Could you check a few things on this model? Use its own coordinates, in mm. A direction names the side the tool comes from. Coordinates: 2 decimals unless noted, no trailing zeros. Order: outer loops, then holes, each group sorted by start corner. A loop starts at its lowest first (then second) coordinate and runs counter-clockwise, first axis right, second up. Notation, with made-up numbers: (-13, 63.5) - (-2, 63.5) arc R26 cw to (-2, 93.5) - close; hole circle Ø9 at (19.5, 18). An arc over 180 degrees is marked (long way). One line per item, written item: value. Start each with the question number.
from build123d import *

# Parameters (mm, degrees)
BOSS_EXTRUDE1_DEPTH = 50.8
SKETCH2_R           = 2.54
CUT_EXTRUDE1_DEPTH  = 88.988181024
SKETCH3_R           = 2.54
CUT_EXTRUDE2_DEPTH  = 88.988181024
FILLET1_R           = 6.35
CHAMFER1_SIZE       = 2.54


with BuildPart() as part:
    # Sketch1 → Boss-Extrude1 (new body)
    with BuildSketch(Plane(origin=(0, 0, 0), x_dir=(0, 0, -1), z_dir=(1, 0, 0))):
        Polygon((0, 0), (0, 50.8), (3.175, 50.8), (3.175, 3.175), (50.8, 3.175), (50.8, 0), align=None)
    extrude(amount=BOSS_EXTRUDE1_DEPTH)

    # Sketch2 → Cut-Extrude1 (cut, through all)
    with BuildSketch(Plane.XY):
        with Locations((12.7, 38.1)):
            Circle(SKETCH2_R)
        with Locations((12.7, 15.875)):
            Circle(SKETCH2_R)
        with Locations((38.1, 38.1)):
            Circle(SKETCH2_R)
        with Locations((38.1, 15.875)):
            Circle(SKETCH2_R)
    extrude(amount=-CUT_EXTRUDE1_DEPTH, mode=Mode.SUBTRACT)

    # Sketch3 → Cut-Extrude2 (cut, through all)
    with BuildSketch(Plane.XZ):
        with Locations(Location((38.1, -38.1, 0), (0, 0, 270))):
            Circle(SKETCH3_R)
        with Locations(Location((38.1, -15.875, 0), (0, 0, 270))):
            Circle(SKETCH3_R)
        with Locations(Location((12.7, -38.1, 0), (0, 0, 270))):
            Circle(SKETCH3_R)
        with Locations(Location((12.7, -15.875, 0), (0, 0, 270))):
            Circle(SKETCH3_R)
    extrude(amount=-CUT_EXTRUDE2_DEPTH, mode=Mode.SUBTRACT)

    # Fillet1
    fillet1_edges = [part.edges().sort_by_distance(p)[0] for p in [
        (25.4, 3.175, -3.175),
    ]]
    fillet(fillet1_edges, radius=FILLET1_R)

    # Chamfer1
    chamfer1_edges = [part.edges().sort_by_distance(p)[0] for p in [
        (50.8, 50.8, -1.5875),
        (0, 50.8, -1.5875),
        (0, 1.5875, -50.8),
        (50.8, 1.5875, -50.8),
    ]]
    chamfer(chamfer1_edges, length=CHAMFER1_SIZE)


solid = part.part
Q1. If I drill on L1, parallel to X at y = 1, z = -38; L2, parallel to Y at x = 12.7, z = -2.4 (3 decimals); L3, parallel to Y at x = 22, z = -27.5 (3 decimals), over which ranges is the centre line in solid material (lowest first)?
Q2. I want a section at B-B on y = 38.1. Please give me the cut outline in (x, z) (3 decimals), then the cut area to 3 significant figures.
Q3. I want a section at D-D on x = 23.5. Please give me the cut outline in (y, z) (3 decimals), then the cut area to 3 significant figures.
Q4. I want a section at C-C on x = 38.1. Please give me the cut outline in (y, z) (3 decimals).
Q5. I want a section at A-A on z = -38.1. Please give me the cut outline in (x, y) (3 decimals).
Q6. I'm going to push flat-ended pins straight in: pin 1 (4 mm diameter, centred on x = 26, y = 26.5, fed in from -Z) (3 decimals); pin 2 (3 mm diameter, centred on x = 38.1, y = 15.875, fed in from -Z); pin 3 (12 mm diameter, centred on x = 22, z = -27, fed in from +Y) (3 decimals). Where does each tip first touch, or does it pass through?
Q7. Which directions (+Z, -Z, +X, -X, +Y, -Y) give clear straight access to the entire face, cutting with the end or side of a thin tool? Please do faces 1 (the flat face through (25, 30, -3.175)), 2 (the cylindrical face through (40.618, 1.565, -15.544)).
Q8. We'd pull the mould along Z, two halves only. Please class faces 3 (the flat face through (49.55, 1.61, -49.51)), 4 (the cylindrical face through (15.218, 1.565, -15.544)), 5 (the flat face through (49.55, 49.51, -1.57)), 6 (the flat face through (25, 25, 0)): +Z half, -Z half, draft (parallel to the pull), parting line (faces both ways), or undercut.
Values follow:
1. L1: x = 0 to 10.16, 15.24 to 35.56, 40.64 to 50.8
1. L2: y = 0 to 13.335, 18.415 to 35.56, 40.64 to 50.8
1. L3: y = 0 to 3.175
2. outline: (0, -3.175) - (10.16, -3.175) - (10.16, 0) - (0, 0) - close; (15.24, -3.175) - (35.56, -3.175) - (35.56, 0) - (15.24, 0) - close; (40.64, -3.175) - (50.8, -3.175) - (50.8, 0) - (40.64, 0) - close
2. area: 129 mm^2
3. outline: (0, -50.8) - (3.175, -50.8) - (3.175, -9.525) arc R6.35 cw to (9.525, -3.175) - (50.8, -3.175) - (50.8, 0) - (0, 0) - close
3. area: 321 mm^2
4. outline: (0, -50.8) - (3.175, -50.8) - (3.175, -40.64) - (0, -40.64) - close; (0, -35.56) - (3.175, -35.56) - (3.175, -18.415) - (0, -18.415) - close; (0, -13.335) - (3.175, -13.335) - (3.175, -9.525) arc R6.35 cw to (9.525, -3.175) - (13.335, -3.175) - (13.335, 0) - (0, 0) - close; (18.415, -3.175) - (35.56, -3.175) - (35.56, 0) - (18.415, 0) - close; (40.64, -3.175) - (50.8, -3.175) - (50.8, 0) - (40.64, 0) - close
5. outline: (0, 0) - (10.16, 0) - (10.16, 3.175) - (0, 3.175) - close; (15.24, 0) - (35.56, 0) - (35.56, 3.175) - (15.24, 3.175) - close; (40.64, 0) - (50.8, 0) - (50.8, 3.175) - (40.64, 3.175) - close
6. pin 1: stops at z = -3.175
6. pin 2: passes through
6. pin 3: stops at y = 3.175
7. face 1: -Z, +X, -X, +Y
7. face 2: +Y, -Y
8. face 3: -Z half
8. face 4: undercut
8. face 5: draft
8. face 6: +Z half
